```python
from build123d import *

# Parameters (mm, degrees)
F0_W      = 71.12
F0_H      = 142.24
F1_DEPTH  = 3.81
F2_W      = 63.5
F2_H      = 134.62
F3_DEPTH  = 5.08
F4_W      = 10.16
F4_H      = 2.54
F5_DEPTH  = 5.334
F6_W      = 7.62
F6_H      = 2.54
F7_DEPTH  = 5.334
F8_W      = 7.62
F8_H      = 2.54
F9_DEPTH  = 4.572
F10_W     = 7.62
F10_H     = 2.54
F11_DEPTH = 4.064
F12_W     = 7.62
F12_H     = 2.54
F13_DEPTH = 4.064
F14_W     = 27.94
F14_H     = 12.7
F15_DEPTH = 4.064
F16_R     = 15.24
F17_DEPTH = 4.064
F18_R     = 5.08


with BuildPart() as f1:
    # F0 (on Top) → F1 (new body, symmetric)
    with BuildSketch(Plane.XY):
        with Locations((0, 13.4339)):
            Rectangle(F0_W, F0_H)
    extrude(amount=F1_DEPTH, both=True)

    # F2 (on face) → F3 (cut)
    with BuildSketch(Plane.XY.offset(3.81)):
        with Locations((0.065597, 14.650529)):
            Rectangle(F2_W, F2_H)
    extrude(amount=-F3_DEPTH, mode=Mode.SUBTRACT)

    # F4 (on face) → F5 (cut)
    with BuildSketch(Plane.XZ.offset(57.6861)):
        with Locations((-17.157398, -0.062746)):
            Rectangle(F4_W, F4_H)
        with Locations((16.987846, -0.278907)):
            Rectangle(F4_W, F4_H)
    extrude(amount=-F5_DEPTH, mode=Mode.SUBTRACT)

    # F6 (on face) → F7 (cut)
    with BuildSketch(Plane.XZ.offset(57.6861)):
        with Locations((-0.01244, -0.158032)):
            Rectangle(F6_W, F6_H)
    extrude(amount=-F7_DEPTH, mode=Mode.SUBTRACT)

    # F8 (on face) → F9 (cut)
    with BuildSketch(Plane.YZ.offset(35.56)):
        with Locations((51.784515, 0.018215)):
            Rectangle(F8_W, F8_H)
    extrude(amount=-F9_DEPTH, mode=Mode.SUBTRACT)

    # F10 (on face) → F11 (cut)
    with BuildSketch(Plane(origin=(-35.56, 0, 0), x_dir=(0, -1, 0), z_dir=(-1, 0, 0))):
        with Locations((-68.214123, 0.094177)):
            Rectangle(F10_W, F10_H)
    extrude(amount=-F11_DEPTH, mode=Mode.SUBTRACT)

    # F12 (on face) → F13 (cut)
    with BuildSketch(Plane(origin=(-35.56, 0, 0), x_dir=(0, -1, 0), z_dir=(-1, 0, 0))):
        with Locations((-50.678022, -0.031994)):
            Rectangle(F12_W, F12_H)
        with Locations((-42.283158, -0.031994)):
            Rectangle(F12_W, F12_H)
    extrude(amount=-F13_DEPTH, mode=Mode.SUBTRACT)

    # F14 (on face) → F15 (cut)
    with BuildSketch(Plane(origin=(0, 0, -3.81), x_dir=(1, 0, 0), z_dir=(0, 0, -1))):
        with Locations((17.181641, -75.335267)):
            Rectangle(F14_W, F14_H)
    extrude(amount=-F15_DEPTH, mode=Mode.SUBTRACT)

    # F16 (on face) → F17 (cut)
    with BuildSketch(Plane(origin=(0, 0, -3.81), x_dir=(1, 0, 0), z_dir=(0, 0, -1))):
        with Locations((0, -39.147473)):
            Circle(F16_R)
    extrude(amount=-F17_DEPTH, mode=Mode.SUBTRACT)

    # F18
    f18_edges = [f1.edges().sort_by_distance(p)[0] for p in [
        (35.56, -57.6861, 0),
        (-35.56, -57.6861, 0),
        (-35.56, 84.5539, 0),
        (35.56, 84.5539, 0),
    ]]
    fillet(f18_edges, radius=F18_R)


solid = f1.part
```
CAD build for the part. Positions are in the model's coordinates, mm. A direction names the side the tool comes from. Coordinates: 2 decimals unless noted, no trailing zeros. Write each loop counter-clockwise with the first axis right and the second up, starting at its lowest first coordinate (ties: lowest second). Pieces come first, ordered by that corner, then holes.
(1) Cut at D-D, the plane y = 8.5. List the corners of the cut face in (x, z), and give its area (3 significant figures).
(2) Cut at A-A, the plane x = 0. List the corners of the cut face in (y, z), and give its area (3 significant figures).
(3) Drill centre lines: probe 1 along Y at (x, z) = (-5.5, 2.75); probe 2 along X at (y, z) = (-9, 2.5); probe 3 along Y at (x, z) = (0, -2). Where is each one in solid material? Low to high.
(4) Flat gauge pins, fed straight in: pin 1 (12 mm diameter, centred on x = 20, y = 27.5, fed in from +Z); pin 2 (2 mm diameter, centred on y = -56.5, z = 0, fed in from +X); pin 3 (0.8 mm diameter, centred on x = -34, z = -0.5, fed in from +Y). Where does each tip first touch, or does it go through?
(5) Cut at B-B, the plane x = -25. List the corners of the cut face in (y, z).
(6) 3-axis set-ups, long thin cutter, end or side, ignore diameter. For faces 1 (the face through (-17, -55, -1.333)), 2 (the face through (0, -52.659, 2)), 3 (the face through (-34, 38.473, 0)): which of +Z, -Z, +X, -X, +Y, -Y reach the whole face in a straight line?
(7) Cut at C-C, the plane y = 36.5. List the corners of the cut face in (x, z), and give its area (3 significant figures).
(8) Two-plate mould, pull along Z, no slides. Class faces 4 (the face through (0, 16, -1.27)), 5 (the face through (35.56, 13, 0)), 6 (the face through (34, 55.595, 0)): +Z half, -Z half, draft (parallel to the pull), parting line (faces both ways), or undercut.
Geometry says:
1. outline: (-35.56, -3.81) - (35.56, -3.81) - (35.56, 3.81) - (31.82, 3.81) - (31.82, -1.27) - (-31.68, -1.27) - (-31.68, 3.81) - (-35.56, 3.81) - close
1. area: 219 mm2
2. outline: (-57.69, -3.81) - (23.91, -3.81) - (23.91, -1.27) - (-52.35, -1.27) - (-52.35, -1.43) - (-57.69, -1.43) - close; (-57.69, 1.11) - (-52.66, 1.11) - (-52.66, 3.81) - (-57.69, 3.81) - close; (54.39, -3.81) - (84.55, -3.81) - (84.55, 3.81) - (81.96, 3.81) - (81.96, -1.27) - (54.39, -1.27) - close
2. area: 310 mm2
3. probe 1: y = -57.69 to -52.66, 81.96 to 84.55
3. probe 2: x = -35.56 to -31.68, 31.82 to 35.56
3. probe 3: y = -57.69 to 23.91, 54.39 to 84.55
4. pin 1: stops at z = -1.27
4. pin 2: stops at x = 34.66
4. pin 3: stops at y = 83.48
5. outline: (-57.69, -3.81) - (84.55, -3.81) - (84.55, 3.81) - (81.96, 3.81) - (81.96, -1.27) - (-52.66, -1.27) - (-52.66, 3.81) - (-57.69, 3.81) - close
6. face 1: -Y
6. face 2: +Z
6. face 3: -X
7. outline: (-35.56, -3.81) - (-15.01, -3.81) - (-15.01, -1.27) - (-31.68, -1.27) - (-31.68, 3.81) - (-35.56, 3.81) - close; (15.01, -3.81) - (35.56, -3.81) - (35.56, 3.81) - (31.82, 3.81) - (31.82, -1.27) - (15.01, -1.27) - close
7. area: 143 mm2
8. face 4: +Z half
8. face 5: draft
8. face 6: undercut
